For this review, take the finished solid that the model builds, in its own axes (mm). A direction names the side the tool comes from. Coordinates: 2 decimals unless noted, no trailing zeros. Loops run counter-clockwise (first coordinate to the right, second up) from the corner with the lowest first, then second, coordinate; pieces in that order, holes last. Notation, with made-up numbers: M 6,25.5 L 37,25.5 A24 cw 37,64.5 Z; hole C -12.5,71 d1. An arc over 180 degrees is marked long. Write item = value, one per line.
Autodesk Inventor part; units mm, degrees
ref_plane "YZ Plane" through (0, 0, 0) normal (1, 0, 0) x (0, 1, 0)
ref_plane "XZ Plane" through (0, 0, 0) normal (0, 1, 0) x (-1, 0, 0)
ref_plane "XY Plane" through (0, 0, 0) normal (0, 0, 1) x (1, 0, 0)
sketch "Sketch1" plane through (0, 0, 0) normal (0, 1, 0) x (-1, 0, 0)
  circle A0 centre (0, 0) radius 15.5
  dimension "d0" = 31
extrude "Extrusion1" add sketch "Sketch1" against normal blind 2.4
sketch "Sketch2" plane through (0, 0, 0) normal (0, 1, 0) x (1, 0, 0)
  circle A0 centre (0, 0) radius 6
  dimension "d3" = 12
extrude "Extrusion2" add sketch "Sketch2" along normal blind 5.6
sketch "Sketch3" plane through (0, 0, 0) normal (0, 1, 0) x (1, 0, 0)
  circle A0 centre (0, 0) radius 2.1
  circle A1 centre (7.9999, -7.9999) radius 2.1
  circle A2 centre (7.9999, 7.9999) radius 2.1
  circle A3 centre (-7.9999, 7.9999) radius 2.1
  circle A4 centre (-7.9999, -7.9999) radius 2.1
  circle A5 centre (0, 0) radius 6.1
  circle A6 centre (0, 0) radius 15.4
  point P0 (0, 0)
extrude "Extrusion3" cut sketch "Sketch3" against normal blind 5.6 contours A1 | A2 | A3 | A4
sketch "Sketch4" plane through (0, 5.6, 0) normal (0, 1, 0) x (1, 0, 0)
  point P0 (0, 0)
hole "Hole1" at (0, 5.6, 0) direction (0, -1, 0) diameter 4.5 end through all
fillet "Fillet1" radius 0.2 1 edges at (-6, 0, 0)
chamfer "Chamfer1" distance 0.2 angle 45 4 edges at (15.5, -2.4, 0) (15.5, 0, 0) (-6, 5.6, 0) (0, 5.6, -2.25)
properties part number "08-0005" material "Aluminum 6061"
Q1. Add section D-D (x = 9.5). State how many separate pieces and enclosed holes the cut face has, and give its area (3 significant figures).
Solved:
separate_pieces = 3
enclosed_holes = 0
area = 44.6 mm²
Q2. Add section B-B (z = 0). Write out the cut boundary in (x, y).
Solved:
outline = M -15.5,-2.2 L -15.3,-2.4 L -2.25,-2.4 L -2.25,5.4 L -2.45,5.6 L -5.8,5.6 L -6,5.4 L -6,0.2 A0.2 cw -6.2,0 L -15.3,0 L -15.5,-0.2 Z; M 2.25,-2.4 L 15.3,-2.4 L 15.5,-2.2 L 15.5,-0.2 L 15.3,0 L 6.2,0 A0.2 cw 6,0.2 L 6,5.4 L 5.8,5.6 L 2.45,5.6 L 2.25,5.4 Z
Q3. Add section A-A (x = 0). Write out the cut boundary in (y, z), and give its area (3 significant figures).
Solved:
outline = M -2.4,-15.3 L -2.2,-15.5 L -0.2,-15.5 L 0,-15.3 L 0,-6.2 A0.2 cw 0.2,-6 L 5.4,-6 L 5.6,-5.8 L 5.6,-2.45 L 5.4,-2.25 L -2.4,-2.25 Z; M -2.4,2.25 L 5.4,2.25 L 5.6,2.45 L 5.6,5.8 L 5.4,6 L 0.2,6 A0.2 cw 0,6.2 L 0,15.3 L -0.2,15.5 L -2.2,15.5 L -2.4,15.3 Z
area = 105 mm²
Q4. For pin 1 Ø2 at (y, z) = (-1, 9) entering from -X; pin 2 Ø6.5 at (x, z) = (8, -8) entering from +Y; pin 3 Ø4 at (x, y) = (-9, 1.5) entering from +Z, all flat-tipped, find the tip position at first contact; note any pin that passes through.
Solved:
pin_1 = -13.28
pin_2 = 0
pin_3 = 13.31
Q5. Draft analysis for pull direction X (two halves, no side actions). For faces 1 (the face through (0, -2.4, -3)), 2 (the face through (-10.098, -1.183, -8.092)), 3 (the face through (2.018, -1.186, 15.368)), state which applies: +X half, -X half, draft (parallel to the pull), parting line (faces both ways), or undercut.
Solved:
face_1 = draft
face_2 = undercut
face_3 = parting line
Q6. Add section C-C (y = 4.25). Write out the cut boundary in (x, z).
Solved:
outline = C 0,0 d12; hole C 0,0 d4.5
Q7. For line 1 along Z through (x, y) = (0, 3.75); line 2 along X through (y, z) = (-0.75, 7.5); line 3 along Y through (x, z) = (-5, -9), list the stretches that pass through material, from the lowest coordinate up.
Solved:
line_1 = -6 to -2.25, 2.25 to 6
line_2 = -13.56 to -10.04, -5.96 to 5.96, 10.04 to 13.56
line_3 = -2.4 to 0
Q8. Machinability: for faces 4 (the face through (-7, 0, 0)), 5 (the face through (2.5, 5.6, 1.2)), which of the approach directions +Z, -Z, +X, -X, +Y, -Y give a long, thin tool a straight path to every point of the face, cutting with its end or side? Answer none if there is none.
Solved:
face_4 = +Y
face_5 = +Z, -Z, +X, -X, +Y
